```python
from build123d import *

# Parameters (mm, degrees)
F0_W     = 622.3
F0_H     = 88.9
F1_DEPTH = 19.05
F2_SIZE  = 88.89999
F3_SIZE  = 88.89999


# Not quite as in the source:
# - a fillet or chamfer is up to 0.001 mm smaller than in the source, because OpenCascade refuses the exact size


with BuildPart() as f1:
    # F0 (on Top) → F1 (new body)
    with BuildSketch(Plane.XY):
        with Locations((-221.6517408729, -17.6658927679)):
            Rectangle(F0_W, F0_H)
    extrude(amount=F1_DEPTH)

    # F2 (size 88.9 in the source; OpenCascade refuses exactly that, so slightly less here)
    f2_edges = [f1.edges().sort_by_distance(p)[0] for p in [
        (-532.801741, 26.784107, 9.525),
    ]]
    chamfer(f2_edges, length=F2_SIZE)

    # F3 (size 88.9 in the source; OpenCascade refuses exactly that, so slightly less here)
    f3_edges = [f1.edges().sort_by_distance(p)[0] for p in [
        (89.498259, 26.784107, 9.525),
    ]]
    chamfer(f3_edges, length=F3_SIZE)


solid = f1.part
```
CAD build for the part. Positions are in the model's coordinates, mm. Coordinates: 2 decimals unless noted, no trailing zeros. Write each loop counter-clockwise with the first axis right and the second up, starting at its lowest first coordinate (ties: lowest second). Pieces come first, ordered by that corner, then holes.
(1) Drill centre lines: probe 1 along X at (y, z) = (18.5, 8.75); probe 2 along Y at (x, z) = (32.5, 6.5); probe 3 along X at (y, z) = (-55, 9.5). Where is each one in solid material? Low to high.
(2) Cut at C-C, the plane y = -25. List the corners of the cut face in (x, z).
(3) Cut at B-B, the plane x = -453. List the corners of the cut face in (y, z), and give its area (3 significant figures).
(4) Flat gauge pins, fed straight in: pin 1 (6 mm diameter, centred on y = 13.5, z = 14, fed in from +X); pin 2 (3 mm diameter, centred on x = -458, z = 12, fed in from +Y); pin 3 (1.5 mm diameter, centred on y = -53, z = 16, fed in from +X). Where does each tip first touch, or does it go through?
Geometry says:
1. probe 1: x = -452.19 to 8.88
1. probe 2: y = -62.12 to -5.12
1. probe 3: x = -525.69 to 82.38
2. outline: (-495.69, 0) - (52.38, 0) - (52.38, 19.05) - (-495.69, 19.05) - close
3. outline: (-62.12, 0) - (17.69, 0) - (17.69, 19.05) - (-62.12, 19.05) - close
3. area: 1,520 mm2
4. pin 1: stops at x = 16.88
4. pin 2: stops at y = 14.19
4. pin 3: stops at x = 81.13
